Source: CAD feature listing. Evaluate the final solid. Frame: model axes, mm. Give positions to 0.01 mm unless a question says otherwise; leave off trailing zeros. Order: outer loops, then holes, each group sorted by start corner. A loop starts at its lowest first (then second) coordinate and runs counter-clockwise, first axis right, second up. Notation, with made-up numbers: (23, 25) - (61, 25) arc R16 ccw to (61, 41) - close; hole circle Ø8 at (-18, 29.5). An arc over 180 degrees is marked (long way). Write each question's results on one line, items separated by ' | '. Start each with the question number.
Item 1: Section A-A on x = 0. Output: boundary loops of the cut face in (y, z).
Item 2: Contact query for flat-ended pins moving along their axis: pin 1 Ø10 at (y, z) = (19.5, 37) entering from +X; pin 2 Ø8 at (y, z) = (-5, 39.5) entering from +X; pin 3 Ø8 at (y, z) = (16, 82) entering from -X; pin 4 Ø7 at (x, z) = (0, 84.73) entering from +Y. Output: stop coordinate, or through.
Item 3: Section D-D on z = 16. Output: boundary loops of the cut face in (x, y).
Item 4: Mould query, pull axis Z, two halves, no side actions, for faces 1 (the flat face through (-12, -19, 0)), 2 (the cylindrical face through (5.725, 23.645, 86.534)), 3 (the flat face through (-12, -19, 105.913)). Classes: released by +Z, released by -Z, zero draft, split by the parting line, or undercut.
Item 5: Line query: line 1 along Z through (x, y) = (0, 24.7); line 2 along Y through (x, z) = (0, 28.5); line 3 along X through (y, z) = (18, 95.5). Output: solid intervals per line, ascending.
Item 6: Section C-C on z = 82.5. Output: boundary loops of the cut face in (x, y), and give its area (3 significant figures).
Item 7: Section B-B on y = 0. Output: boundary loops of the cut face in (x, z).
```python
from build123d import *

# Parameters (mm, degrees)
F0_R          = 26.043045
F1_DEPTH      = 105.912507
F2_R          = 26.043045
F3_R          = 22.133915
F5_DEPTH      = 88.553265
F4_R          = 22.133915
F6_DEPTH      = 185.232297
F7_R          = 6.00256
F8_DEPTH      = 38.1
F8_DEPTH_BACK = 38.1


with BuildPart() as f1:
    # F0 (on Top) → F1 (new body)
    with BuildSketch(Plane.XY):
        Circle(F0_R)
    extrude(amount=F1_DEPTH)

    # F2 (on face) + F3 (on face) → F5 (join)
    with BuildSketch(Plane.XY.offset(105.912507)):
        Circle(F2_R)
    with BuildSketch(Plane.XY.offset(105.912507)):
        Circle(F3_R)
    extrude(amount=-F5_DEPTH)

    # F4 (on face) → F6 (cut)
    with BuildSketch(Plane.XY.offset(105.912507)):
        Circle(F4_R)
    extrude(amount=-F6_DEPTH, mode=Mode.SUBTRACT)

    # F7 (on Front) → F8 (cut, two sides)
    with BuildSketch(Plane.XZ) as f8_sk:
        with Locations((0, 84.731072)):
            Circle(F7_R)
    extrude(amount=F8_DEPTH, mode=Mode.SUBTRACT)
    extrude(f8_sk.sketch, amount=-F8_DEPTH_BACK, mode=Mode.SUBTRACT)


solid = f1.part
```
Evaluation:
1) outline: (-26.04, 0) - (-22.13, 0) - (-22.13, 78.73) - (-26.04, 78.73) - close; (-26.04, 90.73) - (-22.13, 90.73) - (-22.13, 105.91) - (-26.04, 105.91) - close; (22.13, 0) - (26.04, 0) - (26.04, 78.73) - (22.13, 78.73) - close; (22.13, 90.73) - (26.04, 90.73) - (26.04, 105.91) - (22.13, 105.91) - close
2) pin 1: stops at x = 21.63 | pin 2: stops at x = 26.02 | pin 3: stops at x = -23.11 | pin 4: passes through
3) outline: circle Ø52.09 at (0, 0); hole circle Ø44.27 at (0, 0)
4) face 1: released by -Z | face 2: undercut | face 3: released by +Z
5) line 1: z = 0 to 78.73, 90.73 to 105.91 | line 2: y = -26.04 to -22.13, 22.13 to 26.04 | line 3: x = -18.82 to -12.88, 12.88 to 18.82
6) outline: (-5.57, -25.44) - (-5.57, -21.42) arc R22.13 cw to (-5.57, 21.42) - (-5.57, 25.44) arc R26.04 ccw to start; (5.57, -25.44) arc R26.04 ccw to (5.57, 25.44) - (5.57, 21.42) arc R22.13 cw to (5.57, -21.42) - close | area: 504 mm^2
7) outline: (-26.04, 0) - (-22.13, 0) - (-22.13, 105.91) - (-26.04, 105.91) - close; (22.13, 0) - (26.04, 0) - (26.04, 105.91) - (22.13, 105.91) - close
